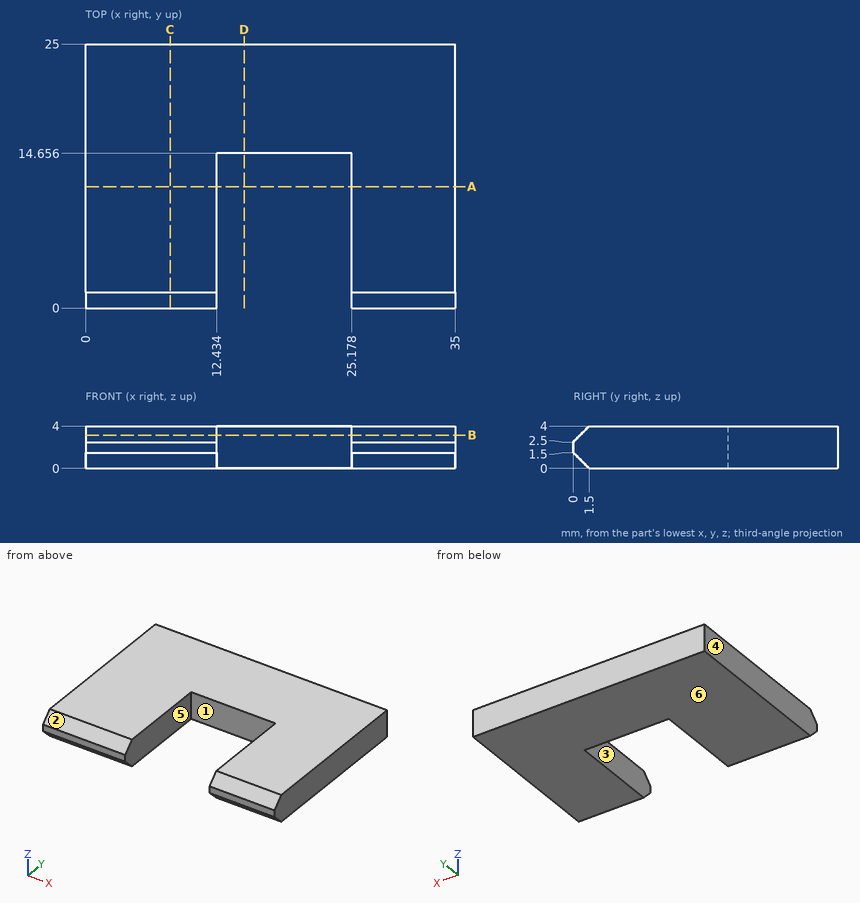
Answer from the drawing. Dimensions are ordinates in mm from the lowest x, y and z of the part. A direction names the side the tool comes from. Give positions to 0.01 mm unless a question says otherwise; leave off trailing zeros. Loops run counter-clockwise (first coordinate to the right, second up) from the corner with the lowest first, then second, coordinate; pieces in that order, holes last.
Item 1: Find the intervals of material crossed by line 1 along X through (y, z) = (6.5, 2.25); line 2 along Y through (x, z) = (14.5, 2.9); line 3 along Z through (x, y) = (6, 1), in increasing order.
Item 2: For the marked faces 5 and 6, determine the directions among +Z, -Z, +X, -X, +Y, -Y from which every point of the face is accessible in a straight line to the end or side of a thin tool.
Item 3: The mould has two halves that part along X. Classify the marked faces 1, 2, 3 and 4: released by +X, released by -X, zero draft, split by the parting line, or undercut.
Item 4: The part is cut by section C-C (x = 8). Write down the section's boundary in (y, z).
Item 5: The part is cut by section D-D (x = 15). Write down the section's boundary in (y, z).
Item 6: The part is cut by section B-B (z = 3.15). Write down the section's boundary in (x, y).
Item 7: The part is cut by section A-A (y = 11.5). Write down the section's boundary in (x, z).
Item 8: Each of these flat-tipped pins is pushed along its axis until it touches: pin 1 Ø5 at (x, y) = (17, 8) entering from +Z (3 decimals); pin 2 Ø1.2 at (x, z) = (21, 2.5) entering from -Y. Where does it stop, or does it pass through?
Taken from the geometry:
1. line 1: x = 0 to 12.43, 25.18 to 35
1. line 2: y = 14.66 to 25
1. line 3: z = 0.5 to 3.5
2. face 5: +Z, -Z, -Y
2. face 6: -Z, +X, -X, +Y, -Y
3. face 1: undercut
3. face 2: zero draft
3. face 3: undercut
3. face 4: released by -X
4. outline: (0, 1.5) - (1.5, 0) - (25, 0) - (25, 4) - (1.5, 4) - (0, 2.5) - close
5. outline: (14.66, 0) - (25, 0) - (25, 4) - (14.66, 4) - close
6. outline: (0, 0.65) - (12.43, 0.65) - (12.43, 14.66) - (25.18, 14.66) - (25.18, 0.65) - (35, 0.65) - (35, 25) - (0, 25) - close
7. outline: (0, 0) - (12.43, 0) - (12.43, 4) - (0, 4) - close; (25.18, 0) - (35, 0) - (35, 4) - (25.18, 4) - close
8. pin 1: passes through
8. pin 2: stops at y = 14.66
